Autodesk Inventor part; units mm, degrees
ref_plane "YZ Plane" through (0, 0, 0) normal (1, 0, 0) x (0, 1, 0)
ref_plane "XZ Plane" through (0, 0, 0) normal (0, 1, 0) x (-1, 0, 0)
ref_plane "XY Plane" through (0, 0, 0) normal (0, 0, 1) x (1, 0, 0)
sketch "Sketch1" plane through (0, 0, 0) normal (0, 1, 0) x (-1, 0, 0)
  circle A0 centre (0, 0) radius 40
  dimension "d2" = 80
extrude "Extrusion1" add sketch "Sketch1" along normal blind 1
sketch "Sketch2" plane through (0, 1, 0) normal (0, 1, 0) x (1, 0, 0)
  circle A0 centre (0, 0) radius 3
  dimension "d3" = 6
extrude "Extrusion2" cut sketch "Sketch2" against normal through all
sketch "Sketch3" plane through (0, 1, 0) normal (0, 1, 0) x (1, 0, 0)
  line L0 (4.9497, 4.9497) -> (-4.9497, 4.9497)
  line L1 (-4.9497, 4.9497) -> (-4.9497, -4.9497)
  line L2 (-4.9497, -4.9497) -> (4.9497, -4.9497)
  line L3 (4.9497, -4.9497) -> (4.9497, 4.9497)
  circle A0 centre (0, 0) radius 3
  line L4 (4.9497, 4.9497) -> (-4.9497, -4.9497) construction
  line L5 (-4.9497, 4.9497) -> (4.9497, -4.9497) construction
  dimension "d6" = 14
  dimension "d7" = 14
  dimension "d8" = 9.8995
  dimension "d9" = 9.8995
hole "Hole1" at (-4.9497, 1, 4.9497) at (-4.9497, 1, -4.9497) at (4.9497, 1, 4.9497) at (4.9497, 1, -4.9497) direction (0, -1, 0) diameter 3.2 end through all
sketch "Sketch4" plane through (0, 0, 0) normal (0, -1, 0) x (1, 0, 0)
  circle A0 centre (4.9497, 4.9497) radius 1.6
  circle A1 centre (-4.9497, 4.9497) radius 1.6
  circle A2 centre (-4.9497, -4.9497) radius 1.6
  circle A3 centre (4.9497, -4.9497) radius 1.6
  circle A4 centre (0, 0) radius 3
  circle A5 centre (0, 0) radius 40
  circle A6 centre (0, 0) radius 40
  line L0 (39.9875, 1) -> (42, 0)
  line L1 (42, 0) -> (39.9875, -1)
  dimension "d18" = 1
  dimension "d19" = 1
  dimension "d20" = 42
extrude "Extrusion3" add sketch "Sketch4" against normal blind 1 contours A5 L0 L1
fillet "Fillet1" radius 1 2 edges at (39.9875, 0.5, -1) (39.9875, 0.5, 1)
equation "\"d8\" = d9"
equation "\"d19\" = d18"
properties part number "IndPlate"
Here's how the part is built. I have some questions about the finished solid (model axes, mm). Coordinates: 2 decimals unless noted, no trailing zeros. Loops run counter-clockwise (first coordinate to the right, second up) from the corner with the lowest first, then second, coordinate; pieces in that order, holes last. Notation, with made-up numbers: M 18.25,41.25 L 59.25,41.25 A7 cw 59.25,50.25 Z; hole C -30.75,47.25 d6. An arc over 180 degrees is marked long. One line per item, written item: value.
1. Imagine slicing it at D-D (z = 21). List the corners of the cut face in (x, y) for me, and give its area (3 significant figures).
Geometry says:
outline: M -34.04,0 L 34.04,0 L 34.04,1 L -34.04,1 Z
area: 68.1 mm2
2. Imagine slicing it at B-B (z = 5.5). List the corners of the cut face in (x, y) for me.
Geometry says:
outline: M -39.62,0 L -6.45,0 L -6.45,1 L -39.62,1 Z; M -3.45,0 L 3.45,0 L 3.45,1 L -3.45,1 Z; M 6.45,0 L 39.62,0 L 39.62,1 L 6.45,1 Z
3. Thinking about a two-plate mould opening in Z: for faces 1 (the cylindrical face through (-3.39, 0.49, -5.3)), 2 (the flat face through (-8, 0, 1)), which applies, +Z half, -Z half, draft (parallel to the pull), parting line (faces both ways), or undercut?
Geometry says:
face 1: undercut
face 2: draft
4. Imagine slicing it at A-A (x = 0). List the corners of the cut face in (y, z) for me, and give its area (3 significant figures).
Geometry says:
outline: M 0,-40 L 1,-40 L 1,-3 L 0,-3 Z; M 0,3 L 1,3 L 1,40 L 0,40 Z
area: 74.0 mm2
5. Imagine slicing it at C-C (y = 0.75). List the corners of the cut face in (x, z) for me.
Geometry says:
outline: M 39.97,-1.59 A1 cw 40.52,-0.73 L 42,0 L 40.52,0.73 A1 cw 39.97,1.59 A40 ccw long Z; hole C -4.95,-4.95 d3.2; hole C -4.95,4.95 d3.2; hole C 0,0 d6; hole C 4.95,-4.95 d3.2; hole C 4.95,4.95 d3.2
6. Please list where these lines run through material, in increasing order: probe 1 along Z at (x, y) = (0, 0.4); probe 2 along Z at (x, y) = (5, 0.9); probe 3 along X at (y, z) = (0.7, 3.5).
Geometry says:
probe 1: z = -40 to -3, 3 to 40
probe 2: z = -39.69 to -6.55, -3.35 to 3.35, 6.55 to 39.69
probe 3: x = -39.85 to -5.63, -4.27 to 4.27, 5.63 to 39.85
